For this review, take the finished solid that the model builds, in its own axes (mm). Face numbers are marked on the shaded views. Round coordinates to 2 decimals unless told otherwise and drop trailing zeros. Order: outer loops, then holes, each group sorted by start corner. A loop starts at its lowest first (then second) coordinate and runs counter-clockwise, first axis right, second up. Notation, with made-up numbers: (28.5, 54) - (85.5, 54) arc R24 cw to (85.5, 85) - close; hole circle Ø2 at (32, 28). An arc over 180 degrees is marked (long way). One line per item, written item: value.
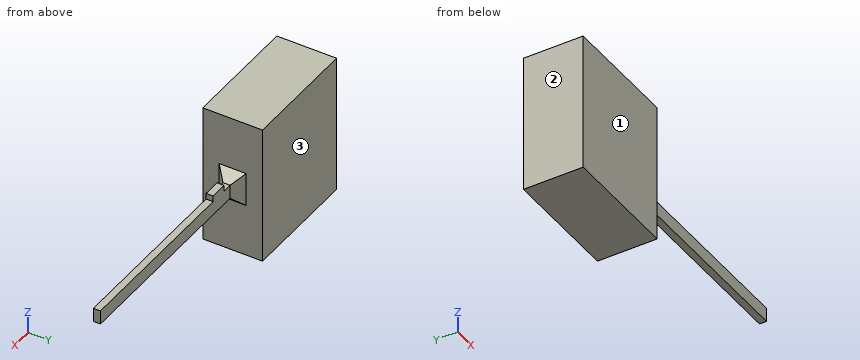
```python
from build123d import *

# Parameters (mm, degrees)
SKETCH1_W           = 6
SKETCH1_H           = 7
BOSS_EXTRUDE1_DEPTH = 3
SKETCH5_W           = 0.698626826
SKETCH5_H           = 0.353353156
BOSS_EXTRUDE3_DEPTH = 0.5
DRAFT1_ANGLE        = 45
SKETCH6_W           = 0.698626826
SKETCH6_H           = 0.353353156
BOSS_EXTRUDE4_DEPTH = 10.5
SKETCH9_W           = 0.888706469
SKETCH9_H           = 0.353353156
BOSS_EXTRUDE5_DEPTH = 0.3


with BuildPart() as part:
    # Sketch1 → Boss-Extrude1 (new body)
    with BuildSketch(Plane(origin=(0, 0, 0), x_dir=(1, 0, 0), z_dir=(0, 1, 0))):
        Rectangle(SKETCH1_W, SKETCH1_H)
    extrude(amount=BOSS_EXTRUDE1_DEPTH)

    # Sketch5 → Boss-Extrude3 (add)
    with BuildSketch(Plane(origin=(3, 0, 0), x_dir=(0, 0, -1), z_dir=(1, 0, 0))):
        with Locations((0, 1.5)):
            Rectangle(SKETCH5_W, SKETCH5_H)
    extrude(amount=BOSS_EXTRUDE3_DEPTH)

    # Draft1
    draft1_faces = [part.faces().sort_by_distance(p)[0] for p in [
        (3.25, 1.323323422, 0),
        (3.25, 1.5, 0.349313413),
        (3.25, 1.676676578, 0),
        (3.25, 1.5, -0.349313413),
    ]]
    draft(draft1_faces, Plane(origin=(3.5, 0, 0), x_dir=(0, 0, 1), z_dir=(1, 0, 0)), DRAFT1_ANGLE)

    # Sketch6 → Boss-Extrude4 (add)
    with BuildSketch(Plane(origin=(3.5, 0, 0), x_dir=(0, 0, -1), z_dir=(1, 0, 0))):
        with Locations((0, 1.5)):
            Rectangle(SKETCH6_W, SKETCH6_H)
    extrude(amount=BOSS_EXTRUDE4_DEPTH)

    # Sketch9 → Boss-Extrude5 (add)
    with BuildSketch(Plane.XY.offset(0.349313413)):
        with Locations((4.427106984, 1.5)):
            Rectangle(SKETCH9_W, SKETCH9_H)
    extrude(amount=BOSS_EXTRUDE5_DEPTH)


solid = part.part
```
Item 1: Take a section at C-C (x = 11). Write out the cut boundary in (y, z), plus the area to 3 significant figures.
Returned:
outline: (1.32, -0.35) - (1.68, -0.35) - (1.68, 0.35) - (1.32, 0.35) - close
area: 0.247 mm^2
Item 2: Take a section at B-B (y = 0.3). Write out the cut boundary in (x, z), plus the area to 3 significant figures.
Returned:
outline: (-3, -3.5) - (3, -3.5) - (3, 3.5) - (-3, 3.5) - close
area: 42.0 mm^2
Item 3: For P1, Ø1.1, axis at x = 10.5, z = 0.5, coming from the -Y side; P2, Ø4, axis at x = 7.5, z = -2.5, coming from the -Y side; P3, Ø3, axis at x = 10.5, z = 0, coming from the +Y side, all flat-tipped, find the tip position at first contact; note any pin that passes through.
Returned:
P1: y = 1.32
P2: through
P3: y = 1.68
Item 4: The part is to be moulded in two halves that separate along Y. For the marked faces 1, 2 and 3, say which applies: +Y half, -Y half, draft (parallel to the pull), parting line (faces both ways), or undercut.
Returned:
face 1: -Y half
face 2: draft
face 3: +Y half
Item 5: Wall thickness on line 1 (X direction, y = 2.65, z = -2.5); line 2 (Y direction, x = 11.5, z = 0); line 3 (Z direction, x = 9.5, y = 1.5): over which ranges is each line inside the solid? List them lowest first.
Returned:
line 1: -3 to 3
line 2: 1.32 to 1.68
line 3: -0.35 to 0.35
Item 6: Take a section at A-A (z = 0). Write out the cut boundary in (x, y).
Returned:
outline: (-3, 0) - (3, 0) - (3, 0.82) - (3.5, 1.32) - (14, 1.32) - (14, 1.68) - (3.5, 1.68) - (3, 2.18) - (3, 3) - (-3, 3) - close
